from build123d import *

# Parameters (mm, degrees)
SKETCH1_W              = 90
SKETCH1_H              = 30.3
BOSS_EXTRUDE1_DEPTH    = 25
SKETCH2_W              = 90
SKETCH2_H              = 20.3
F_2020_SLOT_20_3_DEPTH = 20
SKETCH3_R              = 3
CUT_EXTRUDE2_DEPTH     = 99.19923625
SKETCH5_W              = 90
SKETCH5_H              = 5
BOSS_EXTRUDE2_DEPTH    = 9.4
SKETCH6_W              = 90
SKETCH6_H              = 10
BOSS_EXTRUDE3_DEPTH    = 5
SKETCH7_R              = 3
CUT_EXTRUDE4_DEPTH     = 5
LPATTERN1_COUNT        = 3
LPATTERN1_PITCH        = 22.5
LPATTERN2_COUNT        = 3
LPATTERN2_PITCH        = 22.5
SKETCH10_W             = 90
SKETCH10_H             = 20
BOSS_EXTRUDE4_DEPTH    = 2.7
SKETCH11_W             = 4.5
SKETCH11_H             = 20
CUT_EXTRUDE5_DEPTH     = 2.3
LPATTERN3_COUNT        = 8
LPATTERN3_PITCH        = 10
SKETCH12_W             = 90
SKETCH12_H             = 5
DIFFUSER_SLOT_DEPTH    = 5
SKETCH13_W             = 90
SKETCH13_H             = 10
BOSS_EXTRUDE6_DEPTH    = 5
SKETCH14_W             = 54.7
SKETCH14_H             = 100
BOSS_EXTRUDE7_DEPTH    = 5
SKETCH15_W             = 7.7
SKETCH15_H             = 60
SKETCH15_W_2           = 5
BOSS_EXTRUDE8_DEPTH    = 20
SKETCH16_W             = 5
SKETCH16_H             = 75
BOSS_EXTRUDE9_DEPTH    = 5
SKETCH17_W             = 20
SKETCH17_H             = 25
CUT_EXTRUDE6_DEPTH     = 35
SKETCH18_W             = 4.5
SKETCH18_H             = 50
SKETCH18_W_2           = 2.25
CUT_EXTRUDE7_DEPTH     = 2.3
SKETCH19_W             = 5
SKETCH19_H             = 5
BOSS_EXTRUDE10_DEPTH   = 5
SKETCH20_R             = 3
CUT_EXTRUDE8_DEPTH     = 5
SKETCH22_R             = 3
CUT_EXTRUDE9_DEPTH     = 5


with BuildPart() as part:
    # Sketch1 → Boss-Extrude1 (new body)
    with BuildSketch(Plane(origin=(0, 0, 0), x_dir=(1, 0, 0), z_dir=(0, 1, 0))):
        with Locations((45, -15.15)):
            Rectangle(SKETCH1_W, SKETCH1_H)
    extrude(amount=BOSS_EXTRUDE1_DEPTH)

    # Sketch2 → 2020_Slot_20.3 (cut)
    with BuildSketch(Plane(origin=(0, 25, 0), x_dir=(1, 0, 0), z_dir=(0, 1, 0))):
        with Locations((45, -15.15)):
            Rectangle(SKETCH2_W, SKETCH2_H)
    extrude(amount=-F_2020_SLOT_20_3_DEPTH, mode=Mode.SUBTRACT)

    # Sketch3 → Cut-Extrude2 (cut, through all)
    with BuildSketch(Plane(origin=(0, 0, 0), x_dir=(-1, 0, 0), z_dir=(0, -1, 0))):
        with Locations(Location((-22.5, -15, 0), (0, 0, 90))):
            Circle(SKETCH3_R)
    cut_extrude2 = extrude(amount=-CUT_EXTRUDE2_DEPTH, mode=Mode.SUBTRACT)

    # Sketch5 → Boss-Extrude2 (add)
    with BuildSketch(Plane(origin=(0, 0, 0), x_dir=(-1, 0, 0), z_dir=(0, 0, -1))):
        with Locations((-45, 2.5)):
            Rectangle(SKETCH5_W, SKETCH5_H)
    extrude(amount=BOSS_EXTRUDE2_DEPTH)

    # Sketch6 → Boss-Extrude3 (add)
    with BuildSketch(Plane(origin=(0, 0, -9.4), x_dir=(-1, 0, 0), z_dir=(0, 0, -1))):
        with Locations((-45, 5)):
            Rectangle(SKETCH6_W, SKETCH6_H)
    extrude(amount=BOSS_EXTRUDE3_DEPTH)

    # Sketch7 → Cut-Extrude4 (cut)
    with BuildSketch(Plane.XY.offset(30.3)):
        with Locations((22.5, 15)):
            Circle(SKETCH7_R)
    cut_extrude4 = extrude(amount=-CUT_EXTRUDE4_DEPTH, mode=Mode.SUBTRACT)

    # LPattern1: Cut-Extrude4 ×3
    with Locations(*[(i * LPATTERN1_PITCH, 0, 0) for i in range(1, LPATTERN1_COUNT)]):
        add(cut_extrude4, mode=Mode.SUBTRACT)

    # LPattern2: Cut-Extrude2 ×3
    with Locations(*[(i * LPATTERN2_PITCH, 0, 0) for i in range(1, LPATTERN2_COUNT)]):
        add(cut_extrude2, mode=Mode.SUBTRACT)

    # Sketch10 → Boss-Extrude4 (add)
    with BuildSketch(Plane(origin=(0, 0, 0), x_dir=(-1, 0, 0), z_dir=(0, 0, -1))):
        with Locations((-45, 15)):
            Rectangle(SKETCH10_W, SKETCH10_H)
    extrude(amount=BOSS_EXTRUDE4_DEPTH)

    # Sketch11 → Cut-Extrude5 (cut)
    with BuildSketch(Plane(origin=(0, 0, -2.7), x_dir=(-1, 0, 0), z_dir=(0, 0, -1))):
        with Locations((-10, 15)):
            Rectangle(SKETCH11_W, SKETCH11_H)
    cut_extrude5 = extrude(amount=-CUT_EXTRUDE5_DEPTH, mode=Mode.SUBTRACT)

    # LPattern3: Cut-Extrude5 ×8
    with Locations(*[(i * LPATTERN3_PITCH, 0, 0) for i in range(1, LPATTERN3_COUNT)]):
        add(cut_extrude5, mode=Mode.SUBTRACT)

    # Sketch12 → Diffuser_Slot (add)
    with BuildSketch(Plane(origin=(0, 0, -14.4), x_dir=(-1, 0, 0), z_dir=(0, 0, -1))):
        with Locations((-45, 2.5)):
            Rectangle(SKETCH12_W, SKETCH12_H)
    extrude(amount=DIFFUSER_SLOT_DEPTH)

    # Sketch13 → Boss-Extrude6 (add)
    with BuildSketch(Plane(origin=(0, 0, -19.4), x_dir=(-1, 0, 0), z_dir=(0, 0, -1))):
        with Locations((-45, 5)):
            Rectangle(SKETCH13_W, SKETCH13_H)
    extrude(amount=BOSS_EXTRUDE6_DEPTH)

    # Sketch14 → Boss-Extrude7 (add)
    with BuildSketch(Plane.ZY):
        with Locations((2.95, 50)):
            Rectangle(SKETCH14_W, SKETCH14_H)
    extrude(amount=BOSS_EXTRUDE7_DEPTH)

    # Sketch15 → Boss-Extrude8 (add)
    with BuildSketch(Plane(origin=(0, 0, 0), x_dir=(0, 0, -1), z_dir=(1, 0, 0))):
        with Locations((-1.15, 55)):
            Rectangle(SKETCH15_W, SKETCH15_H)
        with Locations((-27.8, 55)):
            Rectangle(SKETCH15_W_2, SKETCH15_H)
    extrude(amount=BOSS_EXTRUDE8_DEPTH)

    # Sketch16 → Boss-Extrude9 (add)
    with BuildSketch(Plane(origin=(0, 0, 0), x_dir=(0, 0, -1), z_dir=(1, 0, 0))):
        with Locations((11.9, 47.5)):
            Rectangle(SKETCH16_W, SKETCH16_H)
        with Locations((21.9, 47.5)):
            Rectangle(SKETCH16_W, SKETCH16_H)
    extrude(amount=BOSS_EXTRUDE9_DEPTH)

    # Sketch17 → Cut-Extrude6 (cut)
    with BuildSketch(Plane.XY.offset(30.3)):
        with Locations((10, 87.5)):
            Rectangle(SKETCH17_W, SKETCH17_H)
    extrude(amount=-CUT_EXTRUDE6_DEPTH, mode=Mode.SUBTRACT)

    # Sketch18 → Cut-Extrude7 (cut)
    with BuildSketch(Plane(origin=(0, 0, -2.7), x_dir=(-1, 0, 0), z_dir=(0, 0, -1))):
        with Locations((-10, 50)):
            Rectangle(SKETCH18_W, SKETCH18_H)
        with Locations((-18.875, 50)):
            Rectangle(SKETCH18_W_2, SKETCH18_H)
    extrude(amount=-CUT_EXTRUDE7_DEPTH, mode=Mode.SUBTRACT)

    # Sketch19 → Boss-Extrude10 (add)
    with BuildSketch(Plane(origin=(0, 85, 0), x_dir=(1, 0, 0), z_dir=(0, 1, 0))):
        with Locations((2.5, 21.9)):
            Rectangle(SKETCH19_W, SKETCH19_H)
        with Locations((2.5, 11.9)):
            Rectangle(SKETCH19_W, SKETCH19_H)
    extrude(amount=BOSS_EXTRUDE10_DEPTH)

    # Sketch20 → Cut-Extrude8 (cut)
    with BuildSketch(Plane.XY.offset(30.3)):
        with Locations((10, 60)):
            Circle(SKETCH20_R)
        with Locations((10, 40)):
            Circle(SKETCH20_R)
    extrude(amount=-CUT_EXTRUDE8_DEPTH, mode=Mode.SUBTRACT)

    # Sketch22 → Cut-Extrude9 (cut)
    with BuildSketch(Plane.ZY.offset(5)):
        with Locations((15.3, 60)):
            Circle(SKETCH22_R)
        with Locations((15.3, 40.043901833)):
            Circle(SKETCH22_R)
    extrude(amount=-CUT_EXTRUDE9_DEPTH, mode=Mode.SUBTRACT)


solid = part.part
Geometry: final body of the model. Coordinates: model frame, mm. A direction names the side the tool comes from. Round coordinates to 2 decimals unless told otherwise and drop trailing zeros. Order: outer loops, then holes, each group sorted by start corner. A loop starts at its lowest first (then second) coordinate and runs counter-clockwise, first axis right, second up.
Q1. Section C-C, the plane z = -11.5. Output: boundary loops of the cut face in (x, y).
Result sheet:
outline: (-5, 0) - (90, 0) - (90, 10) - (5, 10) - (5, 90) - (0, 90) - (0, 100) - (-5, 100) - close
Q2. Material intervals for probe 1 along X at (y, z) = (1, 15); probe 2 along Z at (x, y) = (18.5, 16.5); probe 3 along Z at (x, y) = (76.5, 7.5), sorted ascending.
Result sheet:
probe 1: x = -5 to 19.5, 25.5 to 42, 48 to 64.5, 70.5 to 90
probe 2: z = -0.4 to 5, 25.3 to 30.3
probe 3: z = -24.4 to -19.4, -14.4 to -9.4, -2.7 to 5, 25.3 to 30.3
Q3. Section A-A, the plane y = 60. Give the number of separate pieces and of enclosed holes in the cut face, and give its area (3 significant figures).
Result sheet:
separate pieces: 3
enclosed holes: 0
area: 502 mm2
Q4. Access query for faces 5 (the face through (4, 40, -2.7)), 6 (the face through (40, 15, -0.4)), 7 (the face through (65.1, 13.2, 27.8)). Directions: +Z, -Z, +X, -X, +Y, -Y. A direction counts if a zero-diameter tool reaches every point of the face in a straight line with its end or side. Return the directions, or none.
Result sheet:
face 5: +X, +Y
face 6: +Y
face 7: +Z
Q5. Mould query, pull axis Y, two halves, no side actions, for faces 1 (the face through (21.85, 12.07, 27.84)), 2 (the face through (-2.535, 62.974, 14.909)), 3 (the face through (55, 25, 28)), 4 (the face through (35, 15, -2.7)). Classes: released by +Y, released by -Y, zero draft, split by the parting line, or undercut.
Result sheet:
face 1: undercut
face 2: undercut
face 3: released by +Y
face 4: zero draft
Q6. Section B-B, the plane x = 45. Output: boundary loops of the cut face in (y, z), and give its area (4 significant figures).
Result sheet:
outline: (0, -24.4) - (10, -24.4) - (10, -19.4) - (5, -19.4) - (5, -14.4) - (10, -14.4) - (10, -9.4) - (5, -9.4) - (5, -2.7) - (25, -2.7) - (25, 5) - (5, 5) - (5, 12) - (0, 12) - close; (0, 18) - (5, 18) - (5, 25.3) - (12, 25.3) - (12, 30.3) - (0, 30.3) - close; (18, 25.3) - (25, 25.3) - (25, 30.3) - (18, 30.3) - close
area: 517.5 mm2
Q7. Section D-D, the plane y = 26.5. Output: boundary loops of the cut face in (x, z), and give its area (3 significant figures).
Result sheet:
outline: (-5, -24.4) - (5, -24.4) - (5, -19.4) - (0, -19.4) - (0, -14.4) - (5, -14.4) - (5, -9.4) - (0, -9.4) - (0, -2.7) - (7.75, -2.7) - (7.75, -0.4) - (12.25, -0.4) - (12.25, -2.7) - (17.75, -2.7) - (17.75, -0.4) - (20, -0.4) - (20, 5) - (0, 5) - (0, 25.3) - (20, 25.3) - (20, 30.3) - (-5, 30.3) - close
area: 562 mm2
Q8. Pin query (flat end, axial travel): pin 1 (2 mm diameter, centred on x = 9, y = 49.5, fed in from -Z); pin 2 (5 mm diameter, centred on x = 71, y = 20, fed in from -Z); pin 3 (2 mm diameter, centred on x = 31.5, z = 9.5, fed in from +Y). Return the tip coordinate at first contact, or that it passes through.
Result sheet:
pin 1: stops at z = -0.4
pin 2: stops at z = -2.7
pin 3: stops at y = 5
